Geometry: final body of the model. Coordinates: model frame, mm. A direction names the side the tool comes from. Coordinates: 2 decimals unless noted, no trailing zeros. Order: outer loops, then holes, each group sorted by start corner. A loop starts at its lowest first (then second) coordinate and runs counter-clockwise, first axis right, second up. Notation, with made-up numbers: (85, -3.5) - (113, -3.5) arc R11 cw to (113, 9.5) - close; hole circle Ø4 at (72.25, -20.5). An arc over 180 degrees is marked (long way). Use one line per item in the form item = value. Start each with the question number.
```python
from build123d import *

# Parameters (mm, degrees)
F0_W     = 60
F0_H     = 60
F1_DEPTH = 5
F2_R     = 25
F3_DEPTH = 2
F4_R     = 10
F5_W     = 6
F5_H     = 3
F5_W_2   = 3
F5_H_2   = 6
F6_DEPTH = 25


with BuildPart() as f1:
    # F0 (on Top) → F1 (new body)
    with BuildSketch(Plane.XY):
        Rectangle(F0_W, F0_H)
    extrude(amount=F1_DEPTH)

    # F2 (on face) → F3 (cut)
    with BuildSketch(Plane.XY.offset(5)):
        Circle(F2_R)
    extrude(amount=-F3_DEPTH, mode=Mode.SUBTRACT)

    # F4
    f4_edges = [f1.edges().sort_by_distance(p)[0] for p in [
        (-30, 30, 2.5),
        (30, 30, 2.5),
        (30, -30, 2.5),
        (-30, -30, 2.5),
    ]]
    fillet(f4_edges, radius=F4_R)

    # F5 (on face) → F6 (cut)
    with BuildSketch(Plane.XY.offset(3)):
        with Locations((-15.041312, -0.136277)):
            Rectangle(F5_W, F5_H)
        with Locations((-0.136277, 15.041312)):
            Rectangle(F5_W_2, F5_H_2)
        with Locations((0.136277, -15.041312)):
            Rectangle(F5_W_2, F5_H_2)
        with Locations((15.041312, 0.136277)):
            Rectangle(F5_W, F5_H)
    extrude(amount=-F6_DEPTH, mode=Mode.SUBTRACT)


solid = f1.part
```
(1) Cut plane D-D on x = -15. Return the cut outline in (y, z).
(2) Cut plane A-A on y = 0. Return the cut outline in (x, z).
(3) Cut plane C-C on z = 1.95. Return the cut outline in (x, y), plus the area to 3 significant figures.
(4) Set-up query: faces 1 (the flat face through (-15, -1.636, 2)), 2 (the cylindrical face through (26.99, -27.15, 2.54)). Return all of +Z, -Z, +X, -X, +Y, -Y with unobstructed straight access to the full face (end or side cutting, diameter ignored); none if empty.
(5) Material intervals for L1, parallel to Y at x = 0, z = 3.6; L2, parallel to X at y = -14, z = 2.25; L3, parallel to Z at x = 17, y = 3.5, sorted ascending. Write a range as from..to.
(6) Draft query along Y for faces 3 (the flat face through (0, -30, 2)), 4 (the flat face through (-18.041, 0, 2)), 5 (the flat face through (0, 0, 0)). Return one class per face: released by +Y, released by -Y, zero draft, split by the parting line, or undercut.
(7) Contact query for a flat-ended pin moving along its axis: pin 1 Ø12 at (x, y) = (2.5, -1) entering from +Z. Output: stop coordinate, or through.
Check sheet entries:
q1.outline = (-30, 0) - (-1.64, 0) - (-1.64, 3) - (-20, 3) - (-20, 5) - (-30, 5) - close; (1.36, 0) - (30, 0) - (30, 5) - (20, 5) - (20, 3) - (1.36, 3) - close
q2.outline = (-30, 0) - (-18.04, 0) - (-18.04, 3) - (-25, 3) - (-25, 5) - (-30, 5) - close; (-12.04, 0) - (12.04, 0) - (12.04, 3) - (-12.04, 3) - close; (18.04, 0) - (30, 0) - (30, 5) - (25, 5) - (25, 3) - (18.04, 3) - close
q3.outline = (-30, -20) arc R10 ccw to (-20, -30) - (20, -30) arc R10 ccw to (30, -20) - (30, 20) arc R10 ccw to (20, 30) - (-20, 30) arc R10 ccw to (-30, 20) - close; hole (-18.04, -1.64) - (-12.04, -1.64) - (-12.04, 1.36) - (-18.04, 1.36) - close; hole (-1.64, 12.04) - (1.36, 12.04) - (1.36, 18.04) - (-1.64, 18.04) - close; hole (-1.36, -18.04) - (1.64, -18.04) - (1.64, -12.04) - (-1.36, -12.04) - close; hole (12.04, -1.36) - (18.04, -1.36) - (18.04, 1.64) - (12.04, 1.64) - close
q3.area = 3,440 mm^2
q4.face_1 = +Z, -Z
q4.face_2 = +Z, -Z, +X, -Y
q5.L1 = -30..-25, 25..30
q5.L2 = -30..-1.36, 1.64..30
q5.L3 = 0..3
q6.face_3 = released by -Y
q6.face_4 = undercut
q6.face_5 = zero draft
q7.pin_1 = 3
